```python
from build123d import *

# Parameters (mm, degrees)
F0_W     = 24.283833
F0_H     = 76.2
F1_DEPTH = 12.7
F2_DEPTH = 50.8
F3_DEPTH = 12.7
F4_DEPTH = 12.7
F6_DEPTH = 125.884833


with BuildPart() as f1:
    # F0 (on Top) → F1 (new body)
    with BuildSketch(Plane.XY):
        with Locations((-57.507079, 7.448686)):
            Rectangle(F0_W, F0_H)
    extrude(amount=F1_DEPTH)

    # F0 (on Top) → F2 (join)
    with BuildSketch(Plane.XY):
        Polygon((56.234837, 45.548686), (-45.365163, 45.548686), (-45.365163, -30.651314), (56.234837, -30.651314), (56.234837, -5.251314), (56.234837, 20.148686), align=None)
    extrude(amount=F2_DEPTH)

    # F0 (on Top) → F3 (join)
    with BuildSketch(Plane.XY):
        Polygon((81.634837, 45.548686), (56.234837, 45.548686), (56.234837, 20.148686), align=None)
    extrude(amount=F3_DEPTH)

    # F0 (on Top) → F4 (join)
    with BuildSketch(Plane.XY):
        Polygon((56.234837, -5.251314), (56.234837, -30.651314), (81.634837, -30.651314), align=None)
    extrude(amount=F4_DEPTH)

    # F5 (on face) → F6 (cut, through all)
    with BuildSketch(Plane.YZ.offset(56.234837)):
        Polygon((20.148686, 50.8), (-5.251314, 50.8), (7.448686, 38.1), align=None)
    extrude(amount=-F6_DEPTH, mode=Mode.SUBTRACT)


solid = f1.part
```
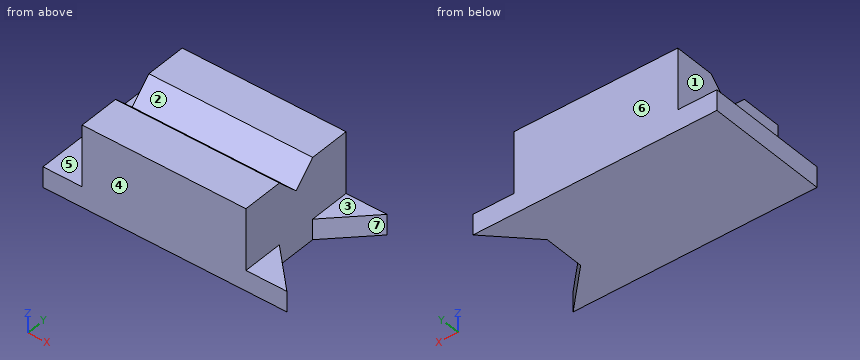
Geometry check sheet. Reference: the model listing, model coordinates, mm. Face numbers are marked on the shaded views. A direction names the side the tool comes from. Round coordinates to 2 decimals unless told otherwise and drop trailing zeros. Loops run counter-clockwise (first coordinate to the right, second up) from the corner with the lowest first, then second, coordinate; pieces in that order, holes last. Notation, with made-up numbers: (7, 68) -> (56, 68) arc R27 ccw to (56, 103) -> close; hole circle Ø10 at (74, 13). An arc over 180 degrees is marked (long way). Use a Markdown table: item, result.
(1) Sectioned sample at C-C (z = 42.5). Enter the section's corners in (x, y).
Calculated:
| item | result |
|---|---|
| outline | (-45.37, -30.65) -> (56.23, -30.65) -> (56.23, 3.05) -> (-45.37, 3.05) -> close; (-45.37, 11.85) -> (56.23, 11.85) -> (56.23, 45.55) -> (-45.37, 45.55) -> close |
(2) Mould release check, pull along Y, two halves, no side actions. Record for the marked faces 4, 5, 6 and 7: released by +Y, released by -Y, zero draft, split by the parting line, or undercut.
Calculated:
| item | result |
|---|---|
| face 4 | released by -Y |
| face 5 | zero draft |
| face 6 | released by +Y |
| face 7 | undercut |
(3) Scan lines: probe 1 along X at (y, z) = (-11.5, 19); probe 2 along Y at (x, z) = (51.5, 45.5); probe 3 along Z at (x, y) = (-48.5, -22.5). Record each from-to range of solid material in increasing order.
Calculated:
| item | result |
|---|---|
| probe 1 | -45.37 to 56.23 |
| probe 2 | -30.65 to 0.05, 14.85 to 45.55 |
| probe 3 | 0 to 12.7 |
(4) Sectioned sample at B-B (x = -20). Enter the section's corners in (y, z).
Calculated:
| item | result |
|---|---|
| outline | (-30.65, 0) -> (45.55, 0) -> (45.55, 50.8) -> (20.15, 50.8) -> (7.45, 38.1) -> (-5.25, 50.8) -> (-30.65, 50.8) -> close |
(5) Set-up check for the marked faces 1, 2 and 3: record each of +Z, -Z, +X, -X, +Y, -Y from which the full face is reachable in a straight line by a thin tool's end or side.
Calculated:
| item | result |
|---|---|
| face 1 | +Z, -X, +Y, -Y |
| face 2 | +Z, +X, -X |
| face 3 | +Z, +X, +Y, -Y |
(6) Sectioned sample at A-A (x = 69). Enter the section's corners in (y, z), then the cut area to 3 significant figures.
Calculated:
| item | result |
|---|---|
| outline | (-30.65, 0) -> (-18.02, 0) -> (-18.02, 12.7) -> (-30.65, 12.7) -> close; (32.91, 0) -> (45.55, 0) -> (45.55, 12.7) -> (32.91, 12.7) -> close |
| area | 321 mm² |
(7) Sectioned sample at D-D (y = -7.5). Enter the section's corners in (x, z), then the cut area to 3 significant figures.
Calculated:
| item | result |
|---|---|
| outline | (-69.65, 0) -> (58.48, 0) -> (58.48, 12.7) -> (56.23, 12.7) -> (56.23, 50.8) -> (-45.37, 50.8) -> (-45.37, 12.7) -> (-69.65, 12.7) -> close |
| area | 5,500 mm² |
(8) Go/stop test with flat-tipped pins: P1, Ø6, axis at y = -11.5, z = 9, coming from the +X side; P2, Ø19.5, axis at x = -56, y = -1, coming from the +Z side; P3, Ø12, axis at y = -7.5, z = 24.5, coming from the +X side. Record where each tip stops, or that it passes through.
Calculated:
| item | result |
|---|---|
| P1 | x = 65.48 |
| P2 | z = 12.7 |
| P3 | x = 56.23 |
